from build123d import *

# Parameters (mm, degrees)
MODEL_R             = 35.6997
MODEL_R_2           = 25.4
MODEL_R_3           = 15.24
BOSS_EXTRUDE2_DEPTH = 15.24
SCALE1_SCALE        = 0.1


with BuildPart() as part:
    # Model → Boss-Extrude2 (new body)
    with BuildSketch(Plane.XY):
        Polygon((683.6156, 410.2862), (683.133, 409.8036), (683.133, 389.7376), (648.0048, 389.7376), (648.0048, 409.702), (647.4968, 410.2862), (550.0116, 410.2862), (550.0116, 1399.2352), (647.4968, 1399.2352), (648.0048, 1399.7432), (648.0048, 1419.7076), (683.133, 1419.7076), (683.133, 1399.8448), (683.641, 1399.3368), (1234.7448, 1399.3368), (1235.202, 1399.8448), (1235.202, 1419.3012), (1269.238, 1419.3012), (1269.238, 1399.7432), (1269.7206, 1399.2352), (1367.3074, 1399.2352), (1366.8248, 409.829), (1269.238, 409.9052), (1269.238, 409.8036), (1269.238, 389.7376), (1234.0844, 389.7376), (1234.0844, 409.8036), (1233.5764, 410.2862), align=None)
        with Locations(Location((958.6214, 472.313, 0), (0, 0, 180))):
            Circle(MODEL_R, mode=Mode.SUBTRACT)
        with Locations(Location((582.0156, 528.8026, 0), (0, 0, 180))):
            Circle(MODEL_R_2, mode=Mode.SUBTRACT)
        with Locations(Location((582.0156, 678.815, 0), (0, 0, 180))):
            Circle(MODEL_R_3, mode=Mode.SUBTRACT)
    extrude(amount=BOSS_EXTRUDE2_DEPTH)


with BuildPart() as part_1:
    # Scale1: scaled about (959.835155039, 908.097861416, 7.62)
    add(part.part.scale(SCALE1_SCALE).moved(Location((863.851639535, 817.288075274, 6.858))))


solid = part_1.part
Can you work these out from the model? Positions are in its coordinate system, mm. Coordinates: 2 decimals unless noted, no trailing zeros. Write each loop counter-clockwise with the first axis right and the second up, starting at its lowest first coordinate (ties: lowest second). Pieces come first, ordered by that corner, then holes. Notation, with made-up numbers: (76, 14.5) -> (102, 14.5) arc R25 ccw to (102, 33.5) -> close; hole circle Ø5 at (43, 39). An arc over 180 degrees is marked (long way). Answer as CSV lines item,"result".
1) If we section it at C-C on z = 7.75: Count the separate pieces of the cut face and the enclosed holes in it, then the cut area to 3 significant figures.
Check result:
separate pieces,"1"
enclosed holes,"3"
area,"8,040 mm²"
2) If I drill on line 1 (Y direction, x = 952, z = 7.75); line 2 (X direction, y = 922.5, z = 7.8); line 3 (X direction, y = 885.5, z = 7.8), over which ranges is the centre line in solid material (lowest first)? Write a range as from..to.
Check result:
line 1,"858.32..957.22"
line 2,"918.85..1000.57"
line 3,"918.85..920.57, 923.54..1000.55"
3) If we mould it in two halves opening along X, with no side actions, what happens to faces 1 (the flat face through (960, 908, 8.382)), 2 (the cylindrical face through (920.88, 872.42, 7.61))? For each: +X half, -X half, draft (parallel to the pull), parting line (faces both ways), or undercut.
Check result:
face 1,"draft"
face 2,"undercut"
4) If we section it at A-A on y = 863: Please give me the cut outline in (x, z).
Check result:
outline,"(918.85, 6.86) -> (956.48, 6.86) -> (956.48, 8.38) -> (918.85, 8.38) -> close; (962.94, 6.86) -> (1000.54, 6.86) -> (1000.54, 8.38) -> (962.94, 8.38) -> close"
5) Will these pins go through, and if not, where does the flat tip stop? P1, Ø0.8, axis at y = 958, z = 8, coming from the -X side; P2, Ø0.5, axis at y = 857, z = 7.5, coming from the +X side; P3, Ø0.8, axis at x = 988.5, z = 7.5, coming from the +Y side; P4, Ø8, axis at x = 922.05, y = 870.17, coming from the +Z side.
Check result:
P1,"x = 928.65"
P2,"x = 990.78"
P3,"y = 959.22"
P4,"z = 8.38"
6) If we section it at B-B on x = 957.5: Please give me the cut outline in (y, z), then the cut area to 3 significant figures.
Check result:
outline,"(858.32, 6.86) -> (861.72, 6.86) -> (861.72, 8.38) -> (858.32, 8.38) -> close; (867.32, 6.86) -> (957.22, 6.86) -> (957.22, 8.38) -> (867.32, 8.38) -> close"
area,"142 mm²"
